```python
from build123d import *

# Parameters (mm, degrees)
BOSS_EXTRUDE1_DEPTH = 3.175


with BuildPart() as part:
    # Sketch1 → Boss-Extrude1 (new body)
    with BuildSketch(Plane.XY):
        with BuildLine():
            Line((18.985, 0), (29.14, 0))
            Line((29.14, 0), (29.14, 14.24))
            Line((29.14, 14.24), (29.14, 17.415))
            Line((29.14, 17.415), (23.312, 17.415))
            Line((23.312, 17.415), (23.312, 14.24))
            Line((23.312, 14.24), (11.656, 14.24))
            Line((11.656, 14.24), (11.656, 17.415))
            Line((11.656, 17.415), (0, 17.415))
            Line((0, 17.415), (0, 14.24))
            Line((0, 14.24), (0, 0))
            Line((0, 0), (15.985, 0))
            ThreePointArc((15.985, 0), (17.485, 1.5), (18.985, 0))
        make_face()
    extrude(amount=BOSS_EXTRUDE1_DEPTH)

    # Mirror1: part across plane


with BuildPart() as part_1:
    add(part.part)
    add(part.part.mirror(Plane(origin=(0, 0, 3.175), x_dir=(0, 0, 1), z_dir=(0, 1, 0))))

    # Mirror3: part across plane


with BuildPart() as part_2:
    add(part_1.part)
    add(part_1.part.mirror(Plane(origin=(29.14, 14.24, 3.175), x_dir=(0, 0, 1), z_dir=(-1, 0, 0))))


solid = part_2.part
```
Could you check a few things on this model? Use its own coordinates, in mm. A direction names the side the tool comes from. Coordinates: 2 decimals unless noted, no trailing zeros. Write each loop counter-clockwise with the first axis right and the second up, starting at its lowest first coordinate (ties: lowest second). Pieces come first, ordered by that corner, then holes. Notation, with made-up numbers: (-25, -26) - (25, -26) arc R34 cw to (25, 8) - close; hole circle Ø11 at (43.5, -23). An arc over 180 degrees is marked (long way). Use a Markdown table: item, result.
Q1. Imagine slicing it at B-B (z = 1.8). List the corners of the cut face in (x, y) for me (3 decimals).
Geometry check:
| item | result |
|---|---|
| outline | (0, -17.415) - (11.656, -17.415) - (11.656, -14.24) - (23.312, -14.24) - (23.312, -17.415) - (34.968, -17.415) - (34.968, -14.24) - (46.624, -14.24) - (46.624, -17.415) - (58.28, -17.415) - (58.28, 17.415) - (46.624, 17.415) - (46.624, 14.24) - (34.968, 14.24) - (34.968, 17.415) - (23.312, 17.415) - (23.312, 14.24) - (11.656, 14.24) - (11.656, 17.415) - (0, 17.415) - close; hole circle Ø3 at (17.485, 0); hole circle Ø3 at (40.795, 0) |
Q2. I'm going to push a flat-ended pin straight in: pin 1 Ø1.6 at (x, z) = (17, 1.5) entering from +Y. Where does the tip first touch, or does it pass through?
Geometry check:
| item | result |
|---|---|
| pin 1 | stops at y = 14.24 |
Q3. Thinking about a two-plate mould opening in X: for faces 4 (the flat face through (29, 17.415, 2)), 5 (the flat face through (41, 14.24, 2)), which applies, +X half, -X half, draft (parallel to the pull), parting line (faces both ways), or undercut?
Geometry check:
| item | result |
|---|---|
| face 4 | draft |
| face 5 | undercut |
Q4. Please list where these lines run through material, in increasing order: L1, parallel to X at y = -14.5, z = 0.75; L2, parallel to X at y = 0, z = 2.4 (3 decimals); L3, parallel to Y at x = 37, z = 0.55.
Geometry check:
| item | result |
|---|---|
| L1 | x = 0 to 11.66, 23.31 to 34.97, 46.62 to 58.28 |
| L2 | x = 0 to 15.985, 18.985 to 39.295, 42.295 to 58.28 |
| L3 | y = -14.24 to 14.24 |
Q5. Imagine slicing it at A-A (y = 0). List the corners of the cut face in (x, z) for me (3 decimals).
Geometry check:
| item | result |
|---|---|
| outline | (0, 0) - (15.985, 0) - (15.985, 3.175) - (0, 3.175) - close; (18.985, 0) - (39.295, 0) - (39.295, 3.175) - (18.985, 3.175) - close; (42.295, 0) - (58.28, 0) - (58.28, 3.175) - (42.295, 3.175) - close |
Q6. Which directions (+Z, -Z, +X, -X, +Y, -Y) give clear straight access to the entire face, cutting with the end or side of a thin tool? Please do faces 1 (the flat face through (30, 0, 3.175)), 2 (the flat face through (41, -14.24, 2)), 3 (the flat face through (23.312, 16, 2)).
Geometry check:
| item | result |
|---|---|
| face 1 | +Z, +X, -X, +Y, -Y |
| face 2 | +Z, -Z, -Y |
| face 3 | +Z, -Z, +Y |
Q7. Imagine slicing it at C-C (x = 14). List the corners of the cut face in (y, z) for me (3 decimals), and give its area (3 significant figures).
Geometry check:
| item | result |
|---|---|
| outline | (-14.24, 0) - (14.24, 0) - (14.24, 3.175) - (-14.24, 3.175) - close |
| area | 90.4 mm2 |
